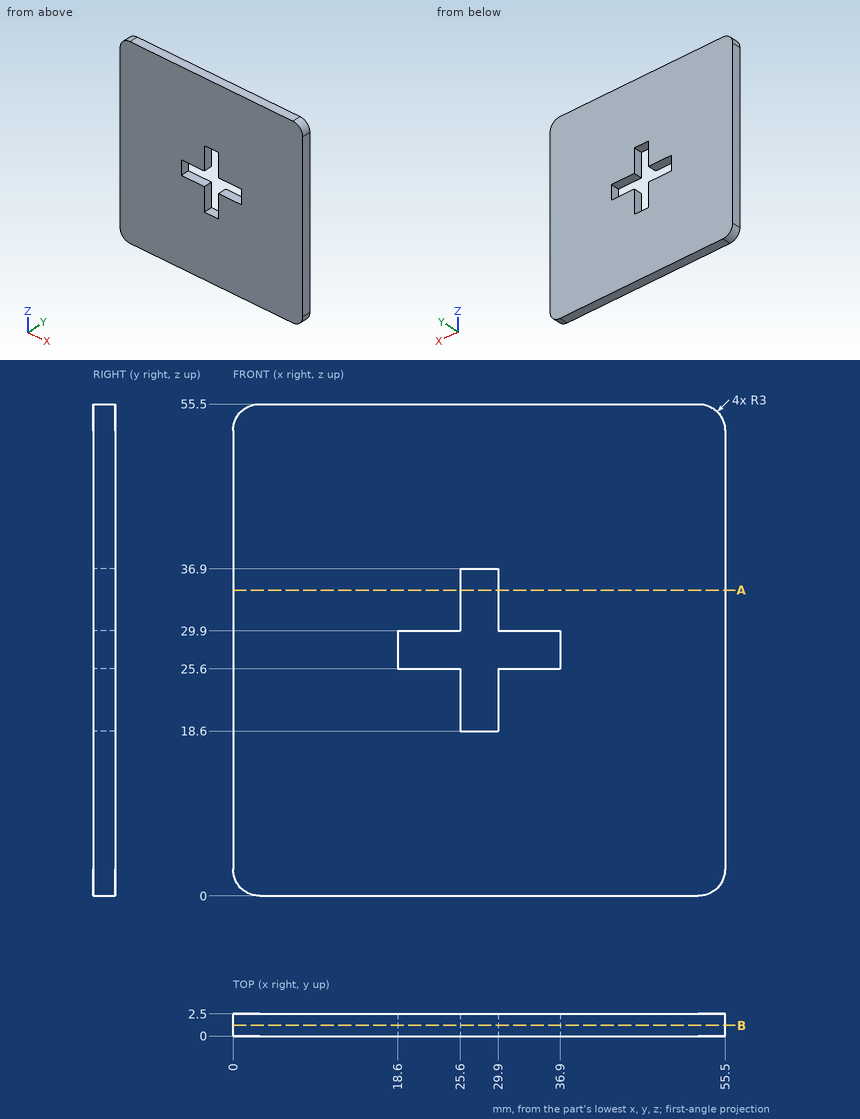
The drawing under review shows one solid part. Ordinate dimensions are in mm from its lowest x, y, z. Coordinates: 2 decimals unless noted, no trailing zeros. Order: outer loops, then holes, each group sorted by start corner. A loop starts at its lowest first (then second) coordinate and runs counter-clockwise, first axis right, second up. Notation, with made-up numbers: (51, 7) - (105, 7) arc R23 cw to (105, 33) - close; hole circle Ø2 at (34.5, 50.5). An arc over 180 degrees is marked (long way). Put each result on its own line as item: value.
1) Take a section at B-B, the plane y = 1.2. Give the boundary of the cut face in (x, z).
Response values:
outline: (0, 3) arc R3 ccw to (3, 0) - (52.5, 0) arc R3 ccw to (55.5, 3) - (55.5, 52.5) arc R3 ccw to (52.5, 55.5) - (3, 55.5) arc R3 ccw to (0, 52.5) - close; hole (18.6, 25.6) - (25.6, 25.6) - (25.6, 18.6) - (29.9, 18.6) - (29.9, 25.6) - (36.9, 25.6) - (36.9, 29.9) - (29.9, 29.9) - (29.9, 36.9) - (25.6, 36.9) - (25.6, 29.9) - (18.6, 29.9) - close
2) Take a section at A-A, the plane z = 34.5. Give the boundary of the cut face in (x, y), and give its area (3 significant figures).
Response values:
outline: (0, 0) - (25.6, 0) - (25.6, 2.5) - (0, 2.5) - close; (29.9, 0) - (55.5, 0) - (55.5, 2.5) - (29.9, 2.5) - close
area: 128 mm²
3) Wall thickness on L1, parallel to Z at x = 33.5, y = 0.25: over which ranges is the line inside the solid? List them lowest first. Write a range as from..to.
Response values:
L1: z = 0..25.6, 29.9..55.5
